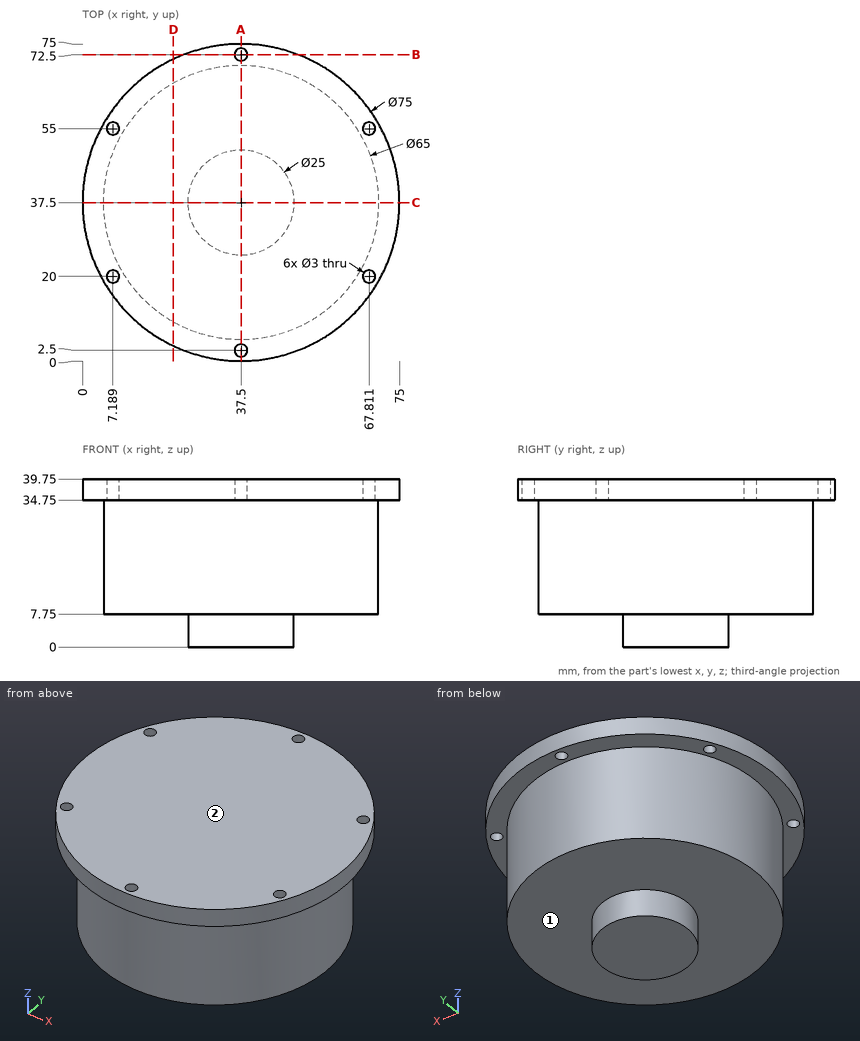
Study the drawing (mm; zero at the part's minimum x, y, z) and answer. A direction names the side the tool comes from. Give positions to 0.01 mm unless a question says otherwise; leave off trailing zeros. Write each loop counter-clockwise with the first axis right and the second up, starting at its lowest first coordinate (ties: lowest second). Pieces come first, ordered by that corner, then holes. Notation, with made-up numbers: M 8,61.25 L 34,61.25 A24 ccw 34,97.25 Z; hole C 64,-7 d8. An arc over 180 degrees is marked long. Put each result on its own line as item: value. Start each with the question number.
1. Each of these flat-tipped pins is pushed along its axis until it touches: pin 1 Ø1.8 at (x, y) = (67.81, 20) entering from +Z; pin 2 Ø10 at (x, z) = (31, 8) entering from +Y; pin 3 Ø2 at (y, z) = (43.5, 9) entering from +X; pin 4 Ø1 at (x, y) = (18, 36.5) entering from -Z. Where does it stop, or does it pass through?
2. Consider line 1 along Y through (x, z) = (37.5, 36.2); line 2 along Z through (x, y) = (46.5, 53); line 3 along X through (y, z) = (37, 26.5). Determine where each line is inside the solid, lowest interval first.
3. The part is cut by section D-D, the plane x = 21.5. Give the vertices of the cut face in (y, z).
4. Which of the six approach directions +Z, -Z, +X, -X, +Y, -Y give full straight-line access (tool end or side, diameter ignored) to the marked faces 1 and 2?
5. The part is cut by section A-A, the plane x = 37.5. Give the vertices of the cut face in (y, z), and give its area (3 significant figures).
6. The part is cut by section B-B, the plane y = 72.5. Give the vertices of the cut face in (x, z).
7. The part is cut by section C-C, the plane y = 37.5. Give the vertices of the cut face in (x, z), and give its area (3 significant figures).
Final values:
1. pin 1: passes through
1. pin 2: stops at y = 69.97
1. pin 3: stops at x = 69.61
1. pin 4: stops at z = 7.75
2. line 1: y = 0 to 1, 4 to 71, 74 to 75
2. line 2: z = 7.75 to 39.75
2. line 3: x = 5 to 70
3. outline: M 3.58,34.75 L 9.21,34.75 L 9.21,7.75 L 65.79,7.75 L 65.79,34.75 L 71.42,34.75 L 71.42,39.75 L 3.58,39.75 Z
4. face 1: -Z
4. face 2: +Z, +X, -X, +Y, -Y
5. outline: M 0,34.75 L 1,34.75 L 1,39.75 L 0,39.75 Z; M 4,34.75 L 5,34.75 L 5,7.75 L 25,7.75 L 25,0 L 50,0 L 50,7.75 L 70,7.75 L 70,34.75 L 71,34.75 L 71,39.75 L 4,39.75 Z; M 74,34.75 L 75,34.75 L 75,39.75 L 74,39.75 Z
5. area: 2,290 mm²
6. outline: M 24.04,34.75 L 36,34.75 L 36,39.75 L 24.04,39.75 Z; M 39,34.75 L 50.96,34.75 L 50.96,39.75 L 39,39.75 Z
7. outline: M 0,34.75 L 5,34.75 L 5,7.75 L 25,7.75 L 25,0 L 50,0 L 50,7.75 L 70,7.75 L 70,34.75 L 75,34.75 L 75,39.75 L 0,39.75 Z
7. area: 2,320 mm²
